```python
from build123d import *

# Parameters (mm, degrees)
SKETCH1_W           = 86
SKETCH1_H           = 66
BOSS_EXTRUDE1_DEPTH = 12
SKETCH2_W           = 81.2
SKETCH2_H           = 61.2
CUT_EXTRUDE1_DEPTH  = 9.6
SKETCH3_R           = 3
BOSS_EXTRUDE2_DEPTH = 4.5
SKETCH4_R           = 1.8
CUT_EXTRUDE2_DEPTH  = 4.5


with BuildPart() as part:
    # Sketch1 → Boss-Extrude1 (new body)
    with BuildSketch(Plane(origin=(0, 0, 0), x_dir=(1, 0, 0), z_dir=(0, 1, 0))):
        Rectangle(SKETCH1_W, SKETCH1_H)
    extrude(amount=BOSS_EXTRUDE1_DEPTH)

    # Sketch2 → Cut-Extrude1 (cut)
    with BuildSketch(Plane.XZ):
        Rectangle(SKETCH2_W, SKETCH2_H)
    extrude(amount=-CUT_EXTRUDE1_DEPTH, mode=Mode.SUBTRACT)

    # Sketch3 → Boss-Extrude2 (add)
    with BuildSketch(Plane.XZ.offset(-9.6)):
        with Locations(Location((-31.5, -21.5, 0), (0, 0, 90))):
            Circle(SKETCH3_R)
        with Locations(Location((31.5, -21.5, 0), (0, 0, 90))):
            Circle(SKETCH3_R)
        with Locations(Location((-31.5, 21.5, 0), (0, 0, 90))):
            Circle(SKETCH3_R)
        with Locations(Location((31.5, 21.5, 0), (0, 0, 90))):
            Circle(SKETCH3_R)
    extrude(amount=BOSS_EXTRUDE2_DEPTH)

    # Sketch4 → Cut-Extrude2 (cut)
    with BuildSketch(Plane.XZ.offset(-9.6)):
        with Locations(Location((-31.5, -21.5, 0), (0, 0, 270))):
            Circle(SKETCH4_R)
        with Locations(Location((31.5, -21.5, 0), (0, 0, 270))):
            Circle(SKETCH4_R)
        with Locations(Location((-31.5, 21.5, 0), (0, 0, 270))):
            Circle(SKETCH4_R)
        with Locations(Location((31.5, 21.5, 0), (0, 0, 270))):
            Circle(SKETCH4_R)
    extrude(amount=-CUT_EXTRUDE2_DEPTH, mode=Mode.SUBTRACT)


solid = part.part
```
Source: CAD feature listing. Evaluate the final solid. Frame: model axes, mm. A direction names the side the tool comes from. Give positions to 0.01 mm unless a question says otherwise; leave off trailing zeros. Write each loop counter-clockwise with the first axis right and the second up, starting at its lowest first coordinate (ties: lowest second). Pieces come first, ordered by that corner, then holes.
1. First-contact query: pin 1 (6.5 mm diameter, centred on x = -30.5, z = -22, fed in from -Y); pin 2 (1.1 mm diameter, centred on x = -30.5, z = 21, fed in from +Y). Flat tips, straight axial feed; report the tip coordinate or a pass-through.
2. Access query for faces 3 (the face through (-32, 5.1, -22)), 4 (the face through (33.285, 10.783, -21.266)), 5 (the face through (-1, 6, -33)). Directions: +Z, -Z, +X, -X, +Y, -Y. A direction counts if a zero-diameter tool reaches every point of the face in a straight line with its end or side. Return the directions, or none.
3. Section query C-C (x = 37). Return the cut outline in (y, z).
4. Section query A-A (y = 8.25). Return the cut outline in (x, z), then the cut area to 3 significant figures.
5. Section query D-D (z = 5.5). Return the cut outline in (x, y).
6. Pull-direction query (X, two-part tool) for faces 1 (the face through (-3, 0, 32)), 2 (the face through (33.285, 10.783, 21.734)); classes: +X half, -X half, draft (parallel to the pull), parting line (faces both ways), or undercut.
7. Section query B-B (y = 1.5). Return the cut outline in (x, z).
8. Material intervals for line 1 along X through (y, z) = (11.5, -21.5); line 2 along X through (y, z) = (9.25, 21.5); line 3 along X through (y, z) = (6.25, 25), sorted ascending.
Output values:
1. pin 1: stops at y = 5.1
1. pin 2: stops at y = 9.6
2. face 3: -Y
2. face 4: +Y
2. face 5: -Z, +X, -X, +Y, -Y
3. outline: (0, -33) - (12, -33) - (12, 33) - (0, 33) - (0, 30.6) - (9.6, 30.6) - (9.6, -30.6) - (0, -30.6) - close
4. outline: (-43, -33) - (43, -33) - (43, 33) - (-43, 33) - close; circle Ø6 at (-31.5, -21.5); circle Ø6 at (-31.5, 21.5); circle Ø6 at (31.5, -21.5); circle Ø6 at (31.5, 21.5); hole (-40.6, -30.6) - (40.6, -30.6) - (40.6, 30.6) - (-40.6, 30.6) - close
4. area: 820 mm2
5. outline: (-43, 0) - (-40.6, 0) - (-40.6, 9.6) - (40.6, 9.6) - (40.6, 0) - (43, 0) - (43, 12) - (-43, 12) - close
6. face 1: draft
6. face 2: undercut
7. outline: (-43, -33) - (43, -33) - (43, 33) - (-43, 33) - close; hole (-40.6, -30.6) - (40.6, -30.6) - (40.6, 30.6) - (-40.6, 30.6) - close
8. line 1: x = -43 to -33.3, -29.7 to 29.7, 33.3 to 43
8. line 2: x = -43 to -40.6, -34.5 to -28.5, 28.5 to 34.5, 40.6 to 43
8. line 3: x = -43 to -40.6, 40.6 to 43
